Input: part model. Units: mm. Frame: model coordinates. Face numbers are marked on the shaded views. A direction names the side the tool comes from. Give positions to 0.01 mm unless a question says otherwise; leave off trailing zeros. Loops run counter-clockwise (first coordinate to the right, second up) from the corner with the lowest first, then second, coordinate; pieces in that order, holes last. Notation, with made-up numbers: M -26,78 L 10,78 A35 ccw 10,113 Z; hole C -23.75,-12 d8. An arc over 180 degrees is marked long. Answer as a JSON object with one key per item and string values. Group by question number.
1) Section query A-A on z = 6.5. Return loops of the section in (x, y).
2) Access query for the marked faces 5 and 6. Directions: +Z, -Z, +X, -X, +Y, -Y. A direction counts if a zero-diameter tool reaches every point of the face in a straight line with its end or side. Return the directions, or none.
3) Ray query, L1, parallel to X at y = 2, z = 6; L2, parallel to Y at x = 12, z = 8.5; L3, parallel to X at y = 6.5, z = 14.25. Return the intervals inside material, ascending.
4) Section query D-D on y = 4. Return loops of the section in (x, z), plus the area to 3 significant figures.
5) First-contact query: P1, Ø1.1, axis at x = -1, y = -16, coming from the +Z side; P2, Ø15.5, axis at x = 4, y = 2.5, coming from the +Z side; P3, Ø0.5, axis at y = -16, z = 13.5, coming from the -X side. Flat tips, straight axial feed; report the tip coordinate or a pass-through.
6) Section query B-B on x = -6. Return loops of the section in (y, z), plus the area to 3 significant figures.
7) Draft query along Y for the marked faces 1, 2, 3 and 4. Return one class per face: +Y half, -Y half, draft (parallel to the pull), parting line (faces both ways), or undercut.
8) Section query C-C on z = 12. Return loops of the section in (x, y), plus the area to 3 significant figures.
from build123d import *

# Parameters (mm, degrees)
PAD_DEPTH       = 18
POCKET_DEPTH    = 16
POCKET001_DEPTH = 5
POCKET002_DEPTH = 5
POCKET003_DEPTH = 4


with BuildPart() as part:
    # Sketch → Pad (new body)
    with BuildSketch(Plane.XY):
        with BuildLine():
            Line((-13.75, -16.5), (13.75, -16.5))
            ThreePointArc((13.75, -16.5), (18.699747, -14.449747), (20.75, -9.5))
            Line((20.75, -9.5), (20.75, 9.5))
            ThreePointArc((20.75, 9.5), (18.699747, 14.449747), (13.75, 16.5))
            Line((13.75, 16.5), (-13.75, 16.5))
            ThreePointArc((-13.75, 16.5), (-18.699747, 14.449747), (-20.75, 9.5))
            Line((-20.75, 9.5), (-20.75, -9.5))
            ThreePointArc((-20.75, -9.5), (-18.699747, -14.449747), (-13.75, -16.5))
        make_face()
    extrude(amount=PAD_DEPTH)

    # Sketch001 (on Face10 of Pad) → Pocket (cut)
    with BuildSketch(Plane.XY.offset(18)):
        with BuildLine():
            Line((-19.25, 11.5), (-19.25, -11.5))
            ThreePointArc((-19.25, -11.5), (-18.078427, -14.328427), (-15.25, -15.5))
            Line((-15.25, -15.5), (15.25, -15.5))
            ThreePointArc((15.25, -15.5), (18.078427, -14.328427), (19.25, -11.5))
            Line((19.25, -11.5), (19.25, 11.5))
            ThreePointArc((19.25, 11.5), (18.078427, 14.328427), (15.25, 15.5))
            Line((15.25, 15.5), (-15.25, 15.5))
            ThreePointArc((-15.25, 15.5), (-18.078427, 14.328427), (-19.25, 11.5))
        make_face()
    extrude(amount=-POCKET_DEPTH, mode=Mode.SUBTRACT)

    # Sketch002 (on Face1 of Pocket) → Pocket001 (cut)
    with BuildSketch(Plane.XZ.offset(16.5)):
        with BuildLine():
            Line((-5.5, 18), (-5.5, 11))
            ThreePointArc((-5.5, 11), (-5.06066, 9.93934), (-4, 9.5))
            Line((-4, 9.5), (2, 9.5))
            ThreePointArc((2, 9.5), (3.06066, 9.93934), (3.5, 11))
            Line((3.5, 11), (3.5, 18))
            ThreePointArc((3.5, 18), (3.06066, 19.06066), (2, 19.5))
            Line((2, 19.5), (-4, 19.5))
            ThreePointArc((-4, 19.5), (-5.06066, 19.06066), (-5.5, 18))
        make_face()
    extrude(amount=-POCKET001_DEPTH, mode=Mode.SUBTRACT)

    # Sketch003 (on Face13 of Pocket001) → Pocket002 (cut)
    with BuildSketch(Plane(origin=(0, 16.5, 0), x_dir=(-1, 0, 0), z_dir=(0, 1, 0))):
        with BuildLine():
            Line((-11.4, 13.5), (-11.4, 11.5))
            ThreePointArc((-11.4, 11.5), (-10.814214, 10.085786), (-9.4, 9.5))
            Line((-9.4, 9.5), (10.6, 9.5))
            ThreePointArc((10.6, 9.5), (12.014214, 10.085786), (12.6, 11.5))
            Line((12.6, 11.5), (12.6, 13.5))
            ThreePointArc((12.6, 13.5), (12.014214, 14.914214), (10.6, 15.5))
            Line((10.6, 15.5), (-9.4, 15.5))
            ThreePointArc((-9.4, 15.5), (-10.814214, 14.914214), (-11.4, 13.5))
        make_face()
    extrude(amount=-POCKET002_DEPTH, mode=Mode.SUBTRACT)

    # Sketch004 (on Face4 of Pocket002) → Pocket003 (cut)
    with BuildSketch(Plane.XY.offset(18)):
        with BuildLine():
            Line((15.2, 9), (15.2, -10))
            ThreePointArc((15.2, -10), (15.63934, -11.06066), (16.7, -11.5))
            Line((16.7, -11.5), (18.7, -11.5))
            ThreePointArc((18.7, -11.5), (19.76066, -11.06066), (20.2, -10))
            Line((20.2, -10), (20.2, 9))
            ThreePointArc((20.2, 9), (19.76066, 10.06066), (18.7, 10.5))
            Line((18.7, 10.5), (16.7, 10.5))
            ThreePointArc((16.7, 10.5), (15.63934, 10.06066), (15.2, 9))
        make_face()
    extrude(amount=-POCKET003_DEPTH, mode=Mode.SUBTRACT)


solid = part.part
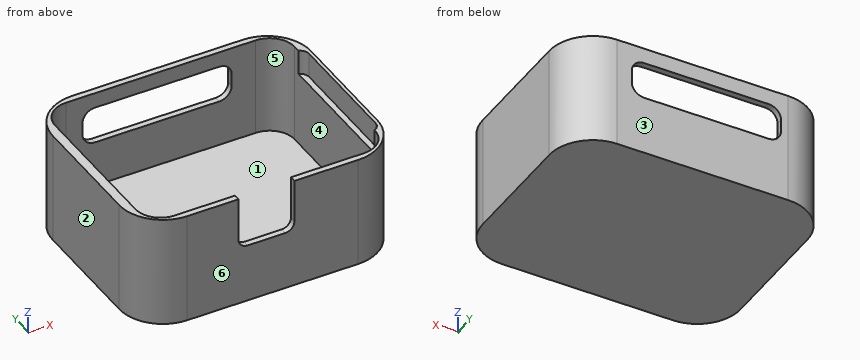
Output:
{
 "1": {"outline": "M -20.75,-9.5 A7 ccw -13.75,-16.5 L 13.75,-16.5 A7 ccw 20.75,-9.5 L 20.75,9.5 A7 ccw 13.75,16.5 L -13.75,16.5 A7 ccw -20.75,9.5 Z; hole M -19.25,-11.5 A4 ccw -15.25,-15.5 L 15.25,-15.5 A4 ccw 19.25,-11.5 L 19.25,11.5 A4 ccw 15.25,15.5 L -15.25,15.5 A4 ccw -19.25,11.5 Z"},
 "2": {"face 5": "+Z", "face 6": "+Z, -Z, +X, -X, -Y"},
 "3": {"L1": "x = -20.75 to -19.25, 19.25 to 20.75", "L2": "y = -16.5 to -15.5, 15.5 to 16.5", "L3": "x = -20.75 to -19.25, 20.2 to 20.75"},
 "4": {"outline": "M -20.75,0 L 20.75,0 L 20.75,18 L 20.2,18 L 20.2,14 L 19.25,14 L 19.25,2 L -19.25,2 L -19.25,18 L -20.75,18 Z", "area": "127 mm^2"},
 "5": {"P1": "stops at z = 9.5", "P2": "stops at z = 2", "P3": "stops at x = -16.9"},
 "6": {"outline": "M -16.5,0 L 16.5,0 L 16.5,9.5 L 15.5,9.5 L 15.5,2 L -15.5,2 L -15.5,18 L -16.5,18 Z; M 15.5,15.5 L 16.5,15.5 L 16.5,18 L 15.5,18 Z", "area": "92.0 mm^2"},
 "7": {"face 1": "undercut", "face 2": "draft", "face 3": "+Y half", "face 4": "undercut"},
 "8": {"outline": "M -20.75,-9.5 A7 ccw -13.75,-16.5 L -5.5,-16.5 L -5.5,-15.5 L -15.25,-15.5 A4 cw -19.25,-11.5 L -19.25,11.5 A4 cw -15.25,15.5 L -12.6,15.5 L -12.6,16.5 L -13.75,16.5 A7 ccw -20.75,9.5 Z; M 3.5,-16.5 L 13.75,-16.5 A7 ccw 20.75,-9.5 L 20.75,9.5 A7 ccw 13.75,16.5 L 11.4,16.5 L 11.4,15.5 L 15.25,15.5 A4 cw 19.25,11.5 L 19.25,-11.5 A4 cw 15.25,-15.5 L 3.5,-15.5 Z", "area": "115 mm^2"}
}
